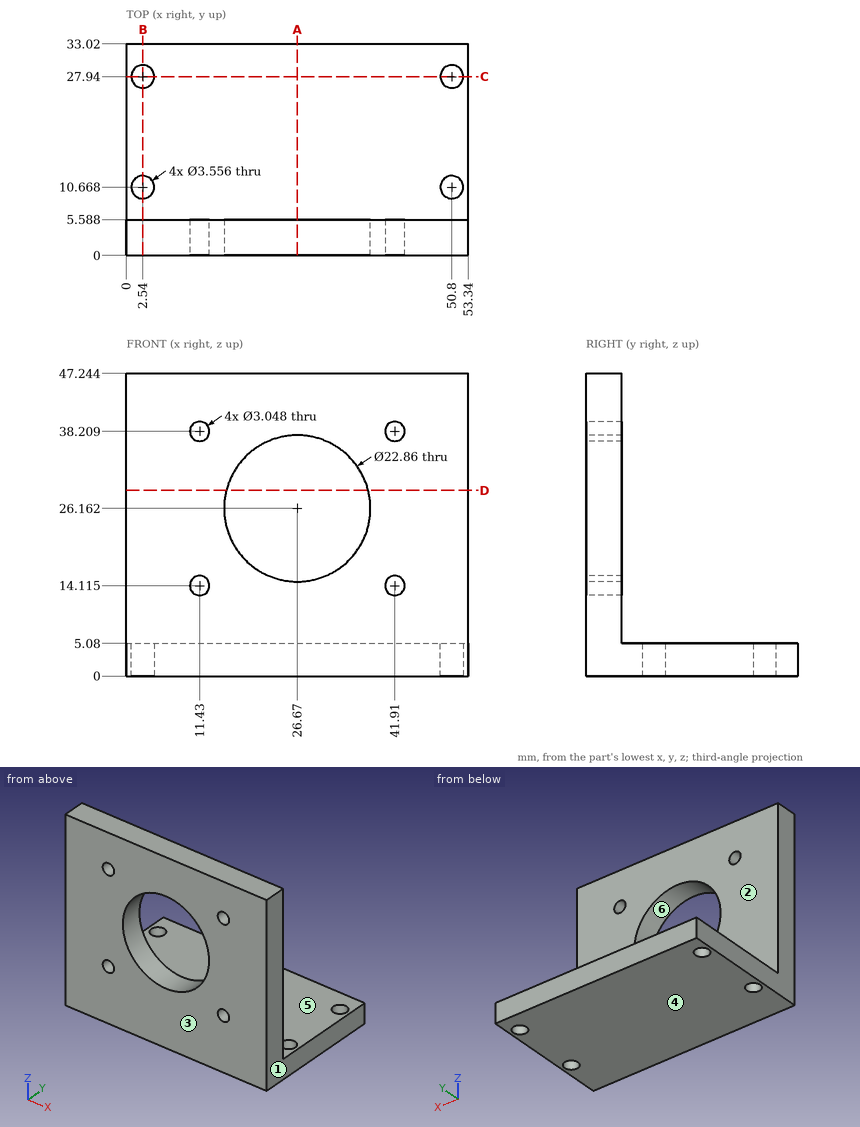
Can you work these out from the drawing? Everything is in mm from the part's minimum corner. A direction names the side the tool comes from. Round coordinates to 2 decimals unless told otherwise and drop trailing zeros. Order: outer loops, then holes, each group sorted by start corner. A loop starts at its lowest first (then second) coordinate and runs counter-clockwise, first axis right, second up. Notation, with made-up numbers: (49.25, -18) - (92.25, -18) arc R31 ccw to (92.25, 18) - close; hole circle Ø3 at (-14, 75). An arc over 180 degrees is marked (long way). Answer in a Markdown table with one row per item.
(1) Which directions (+Z, -Z, +X, -X, +Y, -Y) give clear straight access to the entire face, cutting with the end or side of a thin tool? Please do the marked faces 1 and 2.
From the geometry:
| item | result |
|---|---|
| face 1 | +Z, -Z, +X, +Y, -Y |
| face 2 | +Z, +X, -X, +Y |
(2) Suppose I cut it at A-A, the plane x = 26.67. Please give me the cut outline in (y, z).
From the geometry:
| item | result |
|---|---|
| outline | (0, 0) - (33.02, 0) - (33.02, 5.08) - (5.59, 5.08) - (5.59, 14.73) - (0, 14.73) - close; (0, 37.59) - (5.59, 37.59) - (5.59, 47.24) - (0, 47.24) - close |
(3) Suppose I cut it at C-C, the plane y = 27.94. Please give me the cut outline in (x, z), plus the area to 3 significant figures.
From the geometry:
| item | result |
|---|---|
| outline | (0, 0) - (0.76, 0) - (0.76, 5.08) - (0, 5.08) - close; (4.32, 0) - (49.02, 0) - (49.02, 5.08) - (4.32, 5.08) - close; (52.58, 0) - (53.34, 0) - (53.34, 5.08) - (52.58, 5.08) - close |
| area | 235 mm2 |
(4) Suppose I cut it at D-D, the plane z = 29. Please give me the cut outline in (x, y).
From the geometry:
| item | result |
|---|---|
| outline | (0, 0) - (15.6, 0) - (15.6, 5.59) - (0, 5.59) - close; (37.74, 0) - (53.34, 0) - (53.34, 5.59) - (37.74, 5.59) - close |
(5) If we mould it in two halves opening along Z, with no side actions, what happens to the marked faces 3, 4, 5 and 6? For each: released by +Z, released by -Z, zero draft, split by the parting line, or undercut.
From the geometry:
| item | result |
|---|---|
| face 3 | zero draft |
| face 4 | released by -Z |
| face 5 | released by +Z |
| face 6 | undercut |
(6) For P1, Ø5, axis at x = 11.43, z = 14.12, coming from the +Y side; P2, Ø2, axis at x = 18.5, y = 28, coming from the +Z side, each with a flat end and sliding along its axis, tell me the tip position at first contact or that it passes through.
From the geometry:
| item | result |
|---|---|
| P1 | stops at y = 5.59 |
| P2 | stops at z = 5.08 |
(7) Suppose I cut it at B-B, the plane x = 2.54. Please give me the cut outline in (y, z).
From the geometry:
| item | result |
|---|---|
| outline | (0, 0) - (8.89, 0) - (8.89, 5.08) - (5.59, 5.08) - (5.59, 47.24) - (0, 47.24) - close; (12.45, 0) - (26.16, 0) - (26.16, 5.08) - (12.45, 5.08) - close; (29.72, 0) - (33.02, 0) - (33.02, 5.08) - (29.72, 5.08) - close |
(8) Please list where these lines run through material, in increasing order: L1, parallel to Z at x = 41.91, y = 3.4 (3 decimals); L2, parallel to Y at x = 50.8, z = 3.4; L3, parallel to Z at x = 11, y = 1. Write a range as from..to.
From the geometry:
| item | result |
|---|---|
| L1 | z = 0..12.591, 15.639..36.685, 39.733..47.244 |
| L2 | y = 0..8.89, 12.45..26.16, 29.72..33.02 |
| L3 | z = 0..12.65, 15.58..36.75, 39.67..47.24 |
